Can you work these out from the model? Positions are in its coordinate system, mm. Face numbers are marked on the shaded views. Give positions to 0.01 mm unless a question says otherwise; leave off trailing zeros. Loops run counter-clockwise (first coordinate to the right, second up) from the corner with the lowest first, then second, coordinate; pieces in that order, holes last. Notation, with made-up numbers: (59.25, 75) -> (111.25, 75) arc R19 cw to (111.25, 98) -> close; hole circle Ø3 at (-30, 39). An arc over 180 degrees is marked (long way). Use CSV: the item, a comma, the result in double quotes.
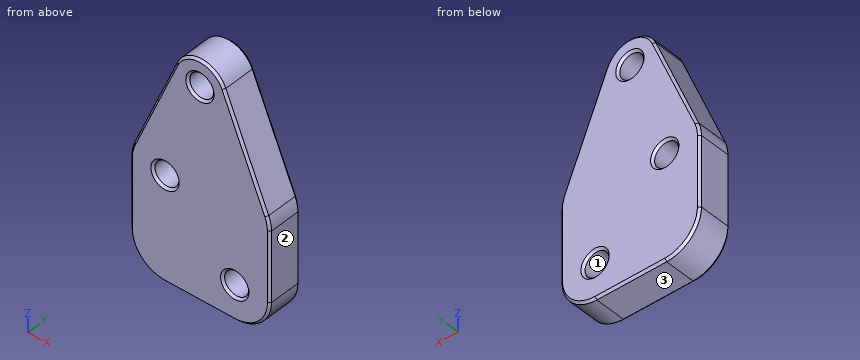
from build123d import *

# Parameters (mm, degrees)
SKETCH1_R           = 2.1828125
BOSS_EXTRUDE1_DEPTH = 6.35
CHAMFER1_SIZE       = 0.396875


with BuildPart() as part:
    # Sketch1 → Boss-Extrude1 (new body)
    with BuildSketch(Plane(origin=(0, 0, 0), x_dir=(1, 0, 0), z_dir=(0, 1, 0))):
        with BuildLine():
            Line((-12.7, 19.05), (-12.7, 31.75))
            ThreePointArc((-12.7, 31.75), (-10.840128061, 36.240128061), (-6.35, 38.1))
            Line((-6.35, 38.1), (6.35, 38.1))
            ThreePointArc((6.35, 38.1), (10.840128061, 36.240128061), (12.7, 31.75))
            Line((12.7, 31.75), (12.7, 19.05))
            ThreePointArc((12.7, 19.05), (12.572860713, 17.785680204), (12.196534001, 16.571988666))
            Line((12.196534001, 16.571988666), (4.384900501, -1.8585085))
            ThreePointArc((4.384900501, -1.8585085), (0, -4.7625), (-4.384900501, -1.8585085))
            Line((-4.384900501, -1.8585085), (-12.196534001, 16.571988666))
            ThreePointArc((-12.196534001, 16.571988666), (-12.572860713, 17.785680204), (-12.7, 19.05))
        make_face()
        Circle(SKETCH1_R, mode=Mode.SUBTRACT)
        with Locations((6.35, 31.75)):
            Circle(SKETCH1_R, mode=Mode.SUBTRACT)
        with Locations((-6.35, 19.05)):
            Circle(SKETCH1_R, mode=Mode.SUBTRACT)
    extrude(amount=BOSS_EXTRUDE1_DEPTH)

    # Chamfer1
    chamfer1_edges = [part.edges().sort_by_distance(p)[0] for p in [
        (8.290717251, 0, -7.356740083),
        (0, 0, 4.7625),
        (-8.290717251, 0, -7.356740083),
        (-12.572860713, 0, -17.785680204),
        (-12.7, 0, -25.4),
        (-10.840128061, 0, -36.240128061),
        (0, 0, -38.1),
        (10.840128061, 6.35, -36.240128061),
        (10.840128061, 0, -36.240128061),
        (12.7, 0, -25.4),
        (12.572860713, 0, -17.785680204),
        (0, 6.35, -38.1),
        (-10.840128061, 6.35, -36.240128061),
        (-12.7, 6.35, -25.4),
        (-2.1828125, 0, 0),
        (-2.1828125, 6.35, 0),
        (-12.572860713, 6.35, -17.785680204),
        (4.1671875, 0, -31.75),
        (4.1671875, 6.35, -31.75),
        (-8.290717251, 6.35, -7.356740083),
        (-8.5328125, 0, -19.05),
        (-8.5328125, 6.35, -19.05),
        (0, 6.35, 4.7625),
        (8.290717251, 6.35, -7.356740083),
        (12.572860713, 6.35, -17.785680204),
        (12.7, 6.35, -25.4),
    ]]
    chamfer(chamfer1_edges, length=CHAMFER1_SIZE)


solid = part.part
(1) If we section it at C-C, the plane z = 0: Write out the boundary of the cut face in (x, y), then the cut area to 3 significant figures.
Answer sheet:
outline,"(-5.17, 0.4) -> (-4.74, 0) -> (-2.58, 0) -> (-2.18, 0.4) -> (-2.18, 5.95) -> (-2.58, 6.35) -> (-4.74, 6.35) -> (-5.17, 5.95) -> close; (2.18, 0.4) -> (2.58, 0) -> (4.74, 0) -> (5.17, 0.4) -> (5.17, 5.95) -> (4.74, 6.35) -> (2.58, 6.35) -> (2.18, 5.95) -> close"
area,"37.3 mm2"
(2) Will these pins go through, and if not, where does the flat tip stop? pin 1 Ø3 at (y, z) = (4.5, -7) entering from -X; pin 2 Ø5.5 at (x, z) = (6.35, -31.75) entering from +Y; pin 3 Ø3.5 at (x, z) = (-6.35, -19.05) entering from +Y.
Answer sheet:
pin 1,"stops at x = -8.78"
pin 2,"stops at y = 6.35"
pin 3,"passes through"
(3) We'd pull the mould along Z, two halves only. Please class the marked faces 1, 2 and 3: released by +Z, released by -Z, zero draft, split by the parting line, or undercut.
Answer sheet:
face 1,"undercut"
face 2,"zero draft"
face 3,"released by -Z"
(4) If I drill on L1, parallel to X at y = 1.75, z = -19.05; L2, parallel to Z at x = 0, y = 2.5; L3, parallel to X at y = 1.75, z = -31.75, over which ranges is the centre line in solid material (lowest first)? Write a range as from..to.
Answer sheet:
L1,"x = -12.7..-8.53, -4.17..12.7"
L2,"z = -38.1..-2.18, 2.18..4.76"
L3,"x = -12.7..4.17, 8.53..12.7"
(5) If we section it at B-B, the plane y = 2.25: Give the number of separate pieces and of enclosed holes in the cut face, then the cut area to 3 significant figures.
Answer sheet:
separate pieces,"1"
enclosed holes,"3"
area,"808 mm2"
(6) If we section it at A-A, the plane x = 0: Write out the boundary of the cut face in (y, z).
Answer sheet:
outline,"(0, -37.7) -> (0.4, -38.1) -> (5.95, -38.1) -> (6.35, -37.7) -> (6.35, -2.58) -> (5.95, -2.18) -> (0.4, -2.18) -> (0, -2.58) -> close; (0, 2.58) -> (0.4, 2.18) -> (5.95, 2.18) -> (6.35, 2.58) -> (6.35, 4.37) -> (5.95, 4.76) -> (0.4, 4.76) -> (0, 4.37) -> close"
(7) If we section it at D-D, the plane z = -13.5: Write out the boundary of the cut face in (x, y), then the cut area to 3 significant figures.
Answer sheet:
outline,"(-10.89, 0.4) -> (-10.46, 0) -> (10.46, 0) -> (10.89, 0.4) -> (10.89, 5.95) -> (10.46, 6.35) -> (-10.46, 6.35) -> (-10.89, 5.95) -> close"
area,"138 mm2"
